Design review of the part built by this model. Coordinates are the model's own, in mm. Coordinates: 2 decimals unless noted, no trailing zeros. Order: outer loops, then holes, each group sorted by start corner. A loop starts at its lowest first (then second) coordinate and runs counter-clockwise, first axis right, second up. Notation, with made-up numbers: M -35.75,36 L -10.75,36 A14 cw -10.75,41 Z; hole C 51,36 d3. An arc over 180 degrees is marked long. Answer as a JSON object with one key per item and string values.
from build123d import *

# Parameters (mm, degrees)
F1_DEPTH = 3.175


with BuildPart() as f1:
    # F0 (on Top) → F1 (new body)
    with BuildSketch(Plane.XY):
        with BuildLine():
            Line((-25.9162820876, 81.5974989146), (-25.9162820876, 30.7974989146))
            ThreePointArc((-25.9162820876, 30.7974989146), (-22.0493623391, 50.2378172787), (-11.0373065718, 66.7185233989))
            Line((-11.0373065718, 66.7185233989), (-25.9162820876, 81.5974989146))
        make_face()
        with BuildLine():
            ThreePointArc((-25.9162820876, 30.7974989146), (-11.0373065718, -5.1235255697), (24.8837179124, -20.0025010854))
            ThreePointArc((24.8837179124, -20.0025010854), (44.3240362766, -16.135581337), (60.8047423967, -5.1235255697))
            Line((60.8047423967, -5.1235255697), (27.1287819427, 28.5524348843))
            ThreePointArc((27.1287819427, 28.5524348843), (22.6386538822, 28.5524348843), (22.6386538822, 33.0425629449))
            Line((22.6386538822, 33.0425629449), (-11.0373065718, 66.7185233989))
            ThreePointArc((-11.0373065718, 66.7185233989), (-22.0493623391, 50.2378172787), (-25.9162820876, 30.7974989146))
        make_face()
        with BuildLine():
            ThreePointArc((60.8047423967, -5.1235255697), (44.3240362766, -16.135581337), (24.8837179124, -20.0025010854))
            Line((24.8837179124, -20.0025010854), (75.6837179124, -20.0025010854))
            Line((75.6837179124, -20.0025010854), (60.8047423967, -5.1235255697))
        make_face()
        with BuildLine():
            Line((60.8047423967, -5.1235255697), (75.6837179124, -20.0025010854))
            Line((75.6837179124, -20.0025010854), (75.6837179124, 30.7974989146))
            ThreePointArc((75.6837179124, 30.7974989146), (71.816798164, 11.3571805505), (60.8047423967, -5.1235255697))
        make_face()
        with BuildLine():
            Line((27.1287819427, 28.5524348843), (60.8047423967, -5.1235255697))
            ThreePointArc((60.8047423967, -5.1235255697), (71.816798164, 11.3571805505), (75.6837179124, 30.7974989146))
            ThreePointArc((75.6837179124, 30.7974989146), (60.8047423967, 66.7185233989), (24.8837179124, 81.5974989146))
            ThreePointArc((24.8837179124, 81.5974989146), (5.4433995483, 77.7305791662), (-11.0373065718, 66.7185233989))
            Line((-11.0373065718, 66.7185233989), (22.6386538822, 33.0425629449))
            ThreePointArc((22.6386538822, 33.0425629449), (26.0987378102, 33.7308164303), (28.0587179124, 30.7974989146))
            ThreePointArc((28.0587179124, 30.7974989146), (27.8170354282, 29.5824790168), (27.1287819427, 28.5524348843))
        make_face()
        with BuildLine():
            Line((24.8837179124, 81.5974989146), (-25.9162820876, 81.5974989146))
            Line((-25.9162820876, 81.5974989146), (-11.0373065718, 66.7185233989))
            ThreePointArc((-11.0373065718, 66.7185233989), (5.4433995483, 77.7305791662), (24.8837179124, 81.5974989146))
        make_face()
        with BuildLine():
            ThreePointArc((24.8837179124, 81.5974989146), (60.8047423967, 66.7185233989), (75.6837179124, 30.7974989146))
            Line((75.6837179124, 30.7974989146), (75.6837179124, 81.5974989146))
            Line((75.6837179124, 81.5974989146), (24.8837179124, 81.5974989146))
        make_face()
    extrude(amount=F1_DEPTH)


solid = f1.part
1) Add section B-B (y = -8). State the section outline as (x, z) points (3 decimals), and give its area (3 significant figures).
Taken from the geometry:
{"outline": "M -7.909,0 L 75.684,0 L 75.684,3.175 L -7.909,3.175 Z", "area": "265 mm2"}
2) To check wall thickness, follow L1, parallel to Y at x = 27.5, z = 1.75; L2, parallel to Y at x = 27, z = 2.35; L3, parallel to X at y = -6.5, z = 0.8. State the ranges of each line that lie inside material, in increasing order.
Taken from the geometry:
{"L1": "y = -20 to 29, 32.6 to 81.6", "L2": "y = -20 to 28.43, 33.16 to 81.6", "L3": "x = -9.61 to 75.68"}
3) Add section C-C (x = 11). State the section outline as (y, z) points (1 decimal).
Taken from the geometry:
{"outline": "M -18.1,0 L 81.6,0 L 81.6,3.2 L -18.1,3.2 Z"}
